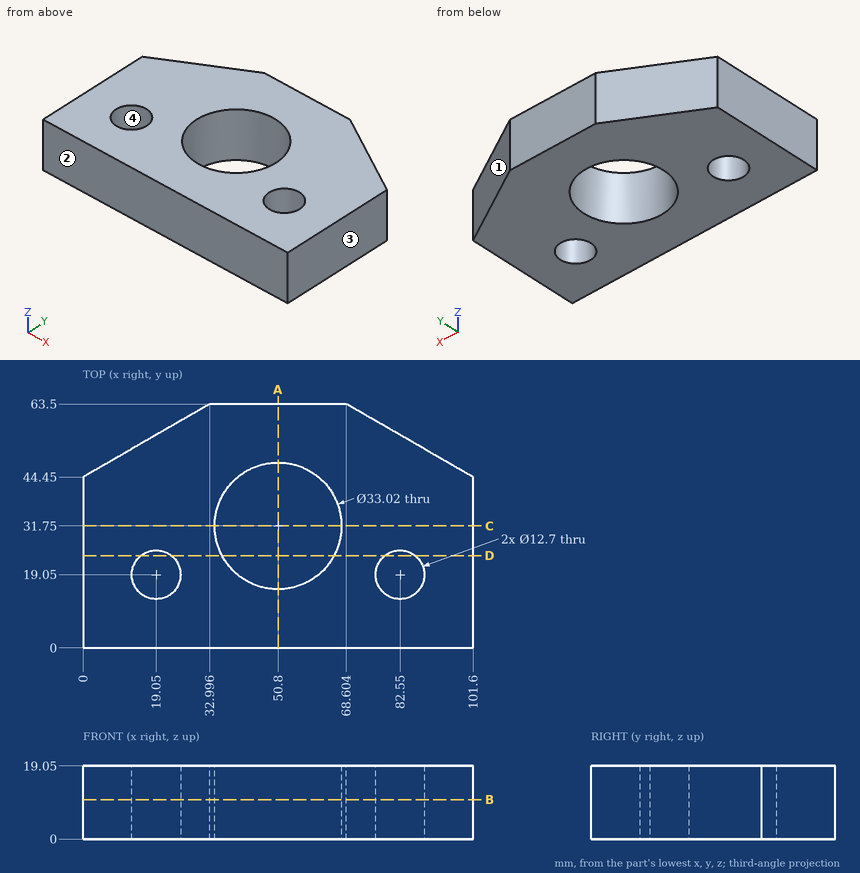
Study the drawing (mm; zero at the part's minimum x, y, z) and answer. Give positions to 0.01 mm unless a question says otherwise; leave off trailing zeros. Order: outer loops, then holes, each group sorted by start corner. A loop starts at its lowest first (then second) coordinate and runs counter-clockwise, first axis right, second up.
1) Find section D-D on y = 24. Write down the section's boundary in (x, z).
Reported:
outline: (0, 0) - (15.07, 0) - (15.07, 19.05) - (0, 19.05) - close; (23.03, 0) - (36.22, 0) - (36.22, 19.05) - (23.03, 19.05) - close; (65.38, 0) - (78.57, 0) - (78.57, 19.05) - (65.38, 19.05) - close; (86.53, 0) - (101.6, 0) - (101.6, 19.05) - (86.53, 19.05) - close
2) Determine the mould class of the marked faces 1, 2, 3 and 4 for opening direction Y: pulls with the +Y half, pulls with the -Y half, needs draft (parallel to the pull), parting line crosses it, or undercut.
Reported:
face 1: pulls with the +Y half
face 2: pulls with the -Y half
face 3: needs draft
face 4: undercut
3) Find section C-C on y = 31.75. Write down the section's boundary in (x, z), then the cut area to 3 significant figures.
Reported:
outline: (0, 0) - (34.29, 0) - (34.29, 19.05) - (0, 19.05) - close; (67.31, 0) - (101.6, 0) - (101.6, 19.05) - (67.31, 19.05) - close
area: 1,310 mm2
4) Find section A-A on x = 50.8. Write down the section's boundary in (y, z), then the cut area to 3 significant figures.
Reported:
outline: (0, 0) - (15.24, 0) - (15.24, 19.05) - (0, 19.05) - close; (48.26, 0) - (63.5, 0) - (63.5, 19.05) - (48.26, 19.05) - close
area: 581 mm2
5) Consider line 1 along X through (y, z) = (32, 10.5); line 2 along Y through (x, z) = (50.8, 10.5); line 3 along Y through (x, z) = (21, 6.5) (1 decimal). Determine where each line is inside the solid, lowest interval first.
Reported:
line 1: x = 0 to 34.29, 67.31 to 101.6
line 2: y = 0 to 15.24, 48.26 to 63.5
line 3: y = 0 to 13, 25.1 to 56.6
6) Given P1, Ø11.5, axis at x = 19.05, y = 19.05, coming from the -Z side; P2, Ø3, axis at x = 25, z = 7, coming from the +Y side; P3, Ø8, axis at x = 86, z = 8.5, coming from the +Y side (1 decimal); P4, Ø6, axis at x = 77.5, z = 7, coming from the +Y side (1 decimal), each flat-ended and moving along its own axis, determine where each tip first touches the part or whether it passes through.
Reported:
P1: passes through
P2: stops at y = 59.75
P3: stops at y = 55.8
P4: stops at y = 60.1
7) Find section B-B on z = 10.25. Give the number of separate pieces and of enclosed holes in the cut face, then the cut area to 3 significant figures.
Reported:
separate pieces: 1
enclosed holes: 3
area: 4,710 mm2
